Build history of the part. All positions in model axes, mm. A direction names the side the tool comes from. Give positions to 0.01 mm unless a question says otherwise; leave off trailing zeros. Order: outer loops, then holes, each group sorted by start corner. A loop starts at its lowest first (then second) coordinate and runs counter-clockwise, first axis right, second up. Notation, with made-up numbers: (35, 13.25) - (77, 13.25) arc R18 cw to (77, 42.25) - close; hole circle Ø10 at (66.5, 64.5). An arc over 180 degrees is marked (long way). Use a Markdown table: item, result.
from build123d import *

# Parameters (mm, degrees)
BOSS_EXTRUDE1_DEPTH      = 16.6
CUT_EXTRUDE1_DEPTH       = 20
BOSS_EXTRUDE2_DEPTH      = 30
BOSS_EXTRUDE2_DEPTH_BACK = 16.6


with BuildPart() as part:
    # Sketch1 → Boss-Extrude1 (new body)
    with BuildSketch(Plane.XY):
        with BuildLine():
            Line((0, 0), (-5, 0))
            ThreePointArc((-5, 0), (-11.010326512, 3.515404103), (-15.3, 9))
            Line((-15.3, 9), (-15.3, 17))
            Line((-15.3, 17), (-8.655870189, 17))
            Line((-8.655870189, 17), (-6.022263631, 19))
            Line((-6.022263631, 19), (0, 19))
            Line((0, 19), (0, 0))
        make_face()
    extrude(amount=BOSS_EXTRUDE1_DEPTH)

    # Sketch2 → Cut-Extrude1 (cut, through all)
    with BuildSketch(Plane.XZ):
        with BuildLine():
            Line((0, 16.6), (-1.7, 16.6))
            ThreePointArc((-1.7, 16.6), (-0.429366175, 12.536153916), (0, 8.3))
            Line((0, 8.3), (0, 16.6))
        make_face()
        with BuildLine():
            Line((0, 0), (0, 8.3))
            ThreePointArc((0, 8.3), (-0.429366175, 4.063846084), (-1.7, 0))
            Line((-1.7, 0), (0, 0))
        make_face()
    extrude(amount=-CUT_EXTRUDE1_DEPTH, mode=Mode.SUBTRACT)

    # Sketch3 → Boss-Extrude2 (add, two sides)
    with BuildSketch(Plane(origin=(0, 29, 0), x_dir=(1, 0, 0), z_dir=(0, 1, 0))) as boss_extrude2_sk:
        with BuildLine():
            Line((-13.4, -1.9), (-2.99735323, -1.9))
            ThreePointArc((-2.99735323, -1.9), (-1.9, -8.3), (-2.99735323, -14.7))
            Line((-2.99735323, -14.7), (-13.4, -14.7))
            Line((-13.4, -14.7), (-13.4, -13.7))
            Line((-13.4, -13.7), (-12.4, -13.7))
            Line((-12.4, -13.7), (-3.71899685, -13.7))
            ThreePointArc((-3.71899685, -13.7), (-2.9, -8.3), (-3.71899685, -2.9))
            Line((-3.71899685, -2.9), (-12.4, -2.9))
            Line((-12.4, -2.9), (-13.4, -2.9))
            Line((-13.4, -2.9), (-13.4, -1.9))
        make_face()
    extrude(amount=BOSS_EXTRUDE2_DEPTH)
    extrude(boss_extrude2_sk.sketch, amount=-BOSS_EXTRUDE2_DEPTH_BACK)


solid = part.part
1) Tool access for faces 1 (the flat face through (-13.4, 38.3, 2.4)), 2 (the cylindrical face through (-1.9, 39.3, 8.2)), 3 (the flat face through (-8, 38, 2.9)), 4 (the flat face through (-7.358, 17.986, 15.637)): list every direction of +Z, -Z, +X, -X, +Y, -Y with a clear straight run to the whole face (end or side of a thin tool).
Computed:
| item | result |
|---|---|
| face 1 | +Z, -Z, -X, +Y |
| face 2 | +X, +Y |
| face 3 | -X, +Y |
| face 4 | +Z, -X, +Y |
2) Wall check: line 1 (Z direction, x = -7.75, y = 20.5); line 2 (Y direction, x = -3.75, z = 7.75); line 3 (Y direction, x = -11.75, z = 8). Give the ranges that are in metal, low to high. Write a range as from..to.
Computed:
| item | result |
|---|---|
| line 1 | z = 1.9..2.9, 13.7..14.7 |
| line 2 | y = 0..19 |
| line 3 | y = 4.2..17 |
3) Pin check, flat tips, straight feed: P1, Ø1.6, axis at x = -5, z = 7, coming from the +Y side; P2, Ø3, axis at x = -3.5, z = 11.5, coming from the +Y side; P3, Ø8.5, axis at x = -10.5, y = 30, coming from the -Z side; P4, Ø1.5, axis at y = 9, z = 13, coming from the +X side. Stop position of each tip, or through.
Computed:
| item | result |
|---|---|
| P1 | stops at y = 19 |
| P2 | stops at y = 59 |
| P3 | stops at z = 1.9 |
| P4 | stops at x = -0.37 |
4) Slice it at A-A (y = 41). Write the cut outline in (x, z).
Computed:
| item | result |
|---|---|
| outline | (-13.4, 1.9) - (-3, 1.9) arc R19.21 ccw to (-3, 14.7) - (-13.4, 14.7) - (-13.4, 13.7) - (-3.72, 13.7) arc R18.21 cw to (-3.72, 2.9) - (-13.4, 2.9) - close |
5) Slice it at B-B (z = 11). Write the cut outline in (x, y), and give its area (3 significant figures).
Computed:
| item | result |
|---|---|
| outline | (-15.3, 9) arc R18.54 ccw to (-5, 0) - (-0.17, 0) - (-0.17, 19) - (-2.09, 19) - (-2.09, 59) - (-3.1, 59) - (-3.1, 19) - (-6.02, 19) - (-8.66, 17) - (-15.3, 17) - close |
| area | 278 mm² |
6) Two-plate mould, pull along Z, no slides. Class faces 5 (the flat face through (-4, 19, 8)), 6 (the flat face through (-9, 38, 13.7)), 7 (the flat face through (-2.5, 59, 7.8)), 8 (the flat face through (-7, 10, 16.6)): +Z half, -Z half, draft (parallel to the pull), parting line (faces both ways), or undercut.
Computed:
| item | result |
|---|---|
| face 5 | undercut |
| face 6 | undercut |
| face 7 | draft |
| face 8 | +Z half |
7) Slice it at D-D (y = 15). Write the cut outline in (x, z).
Computed:
| item | result |
|---|---|
| outline | (-15.3, 0) - (-1.7, 0) arc R21.11 ccw to (-1.7, 16.6) - (-15.3, 16.6) - close |
8) Slice it at C-C (x = -11.25). Write the cut outline in (y, z), and give its area (3 significant figures).
Computed:
| item | result |
|---|---|
| outline | (3.73, 0) - (17, 0) - (17, 1.9) - (59, 1.9) - (59, 2.9) - (17, 2.9) - (17, 13.7) - (59, 13.7) - (59, 14.7) - (17, 14.7) - (17, 16.6) - (3.73, 16.6) - close |
| area | 304 mm² |
